Geometry: final body of the model. Coordinates: model frame, mm. A direction names the side the tool comes from. Give positions to 0.01 mm unless a question says otherwise; leave off trailing zeros. Write each loop counter-clockwise with the first axis right and the second up, starting at its lowest first coordinate (ties: lowest second). Pieces come first, ordered by that corner, then holes.
Q1. Reachability of faces 1 (the flat face through (18, 85, -24)), 2 (the cylindrical face through (56.315, 87.465, -1.201)) from +Z, -Z, +X, -X, +Y, -Y: full face, straight path, thin tool, end or side. Return the list, or none.
Q2. Mould query, pull axis X, two halves, no side actions, for faces 3 (the cylindrical face through (-0.4, 87.5, -52.5)), 4 (the cylindrical face through (-5.961, 44.37, 26.846)), 5 (the flat face through (18, 90, -24)). Classes: +X half, -X half, draft (parallel to the pull), parting line (faces both ways), or undercut.
Q3. Pin query (flat end, axial travel): pin 1 Ø4 at (y, z) = (33.5, -26.5) entering from -X; pin 2 Ø10 at (x, y) = (7.5, 21.5) entering from -Z. Return the tip coordinate at first contact, or that it passes through.
Q4. Section D-D (y = 67.5). Return the cut outline in (x, z).
Q5. Section A-A (z = 0). Return the cut outline in (x, y).
Q6. Section B-B (x = 0). Return the cut outline in (y, z).
Q7. Line query: line 1 (X direction, y = 87.25, z = 0); line 2 (Z direction, x = 0, y = 22). Output: solid intervals per line, ascending.
Q8. Section C-C (z = 13.5). Return the cut outline in (x, y).
from build123d import *

# Parameters (mm, degrees)
SKETCH1_R           = 29.5
SKETCH1_R_2         = 27.5
BOSS_EXTRUDE1_DEPTH = 85
SKETCH2_R           = 4
SKETCH2_R_2         = 27.5
BOSS_EXTRUDE2_DEPTH = 5


with BuildPart() as part:
    # Sketch1 → Boss-Extrude1 (new body)
    with BuildSketch(Plane(origin=(0, 0, 0), x_dir=(1, 0, 0), z_dir=(0, 1, 0))):
        Circle(SKETCH1_R)
        Circle(SKETCH1_R_2, mode=Mode.SUBTRACT)
    extrude(amount=BOSS_EXTRUDE1_DEPTH)

    # Sketch2 → Boss-Extrude2 (add)
    with BuildSketch(Plane(origin=(0, 85, 0), x_dir=(1, 0, 0), z_dir=(0, 1, 0))):
        with BuildLine():
            Line((30, 43.084219849), (65.357142857, 18.46466565))
            ThreePointArc((65.357142857, 18.46466565), (75, 0), (65.357142857, -18.46466565))
            Line((65.357142857, -18.46466565), (30, -43.084219849))
            ThreePointArc((30, -43.084219849), (0, -52.5), (-30, -43.084219849))
            Line((-30, -43.084219849), (-65.357142857, -18.46466565))
            ThreePointArc((-65.357142857, -18.46466565), (-75, 0), (-65.357142857, 18.46466565))
            Line((-65.357142857, 18.46466565), (-30, 43.084219849))
            ThreePointArc((-30, 43.084219849), (0, 52.5), (30, 43.084219849))
        make_face()
        with Locations((52.5, 0)):
            Circle(SKETCH2_R, mode=Mode.SUBTRACT)
        with Locations((-52.5, 0)):
            Circle(SKETCH2_R, mode=Mode.SUBTRACT)
        Circle(SKETCH2_R_2, mode=Mode.SUBTRACT)
    extrude(amount=BOSS_EXTRUDE2_DEPTH)


solid = part.part
Computed:
1. face 1: -Y
1. face 2: +Y, -Y
2. face 3: parting line
2. face 4: undercut
2. face 5: draft
3. pin 1: stops at x = -16.43
3. pin 2: stops at z = -29.39
4. outline: circle Ø59 at (0, 0); hole circle Ø55 at (0, 0)
5. outline: (-75, 85) - (-56.5, 85) - (-56.5, 90) - (-75, 90) - close; (-48.5, 85) - (-29.5, 85) - (-29.5, 0) - (-27.5, 0) - (-27.5, 90) - (-48.5, 90) - close; (27.5, 0) - (29.5, 0) - (29.5, 85) - (48.5, 85) - (48.5, 90) - (27.5, 90) - close; (56.5, 85) - (75, 85) - (75, 90) - (56.5, 90) - close
6. outline: (0, -29.5) - (85, -29.5) - (85, -52.5) - (90, -52.5) - (90, -27.5) - (0, -27.5) - close; (0, 27.5) - (90, 27.5) - (90, 52.5) - (85, 52.5) - (85, 29.5) - (0, 29.5) - close
7. line 1: x = -75 to -56.5, -48.5 to -27.5, 27.5 to 48.5, 56.5 to 75
7. line 2: z = -29.5 to -27.5, 27.5 to 29.5
8. outline: (-70.5, 85) - (-26.23, 85) - (-26.23, 0) - (-23.96, 0) - (-23.96, 90) - (-70.5, 90) - close; (23.96, 0) - (26.23, 0) - (26.23, 85) - (70.5, 85) - (70.5, 90) - (23.96, 90) - close
